Source: three-view drawing plus pictorial views. Frame: mm from the lowest corner of the part. Give positions to 0.01 mm unless a question says otherwise; leave off trailing zeros. Order: outer loops, then holes, each group sorted by start corner. A loop starts at its lowest first (then second) coordinate and runs counter-clockwise, first axis right, second up. Notation, with made-up numbers: (-34.5, 58) - (19.5, 58) arc R9 ccw to (19.5, 72) - close; hole circle Ø3 at (66.5, -13.5). An arc over 180 degrees is marked (long way). Answer in a Markdown table with one row per item. Add a question column.
1. Ray query, line 1 (Y direction, x = 5.25, z = 6); line 2 (Y direction, x = 7.5, z = 7); line 3 (Z direction, x = 6.25, y = 83.75). Return the intervals inside material, ascending. Write a range as [from, to].
2. Contact query for a flat-ended pin moving along its axis: pin 1 (2.5 mm diameter, centred on y = 83.75, z = 6, fed in from +X). Output: stop coordinate, or through.
3. Section query B-B on y = 3.75. Return loops of the section in (x, z), and give its area (3 significant figures).
4. Section query A-A on z = 6. Return loops of the section in (x, y).
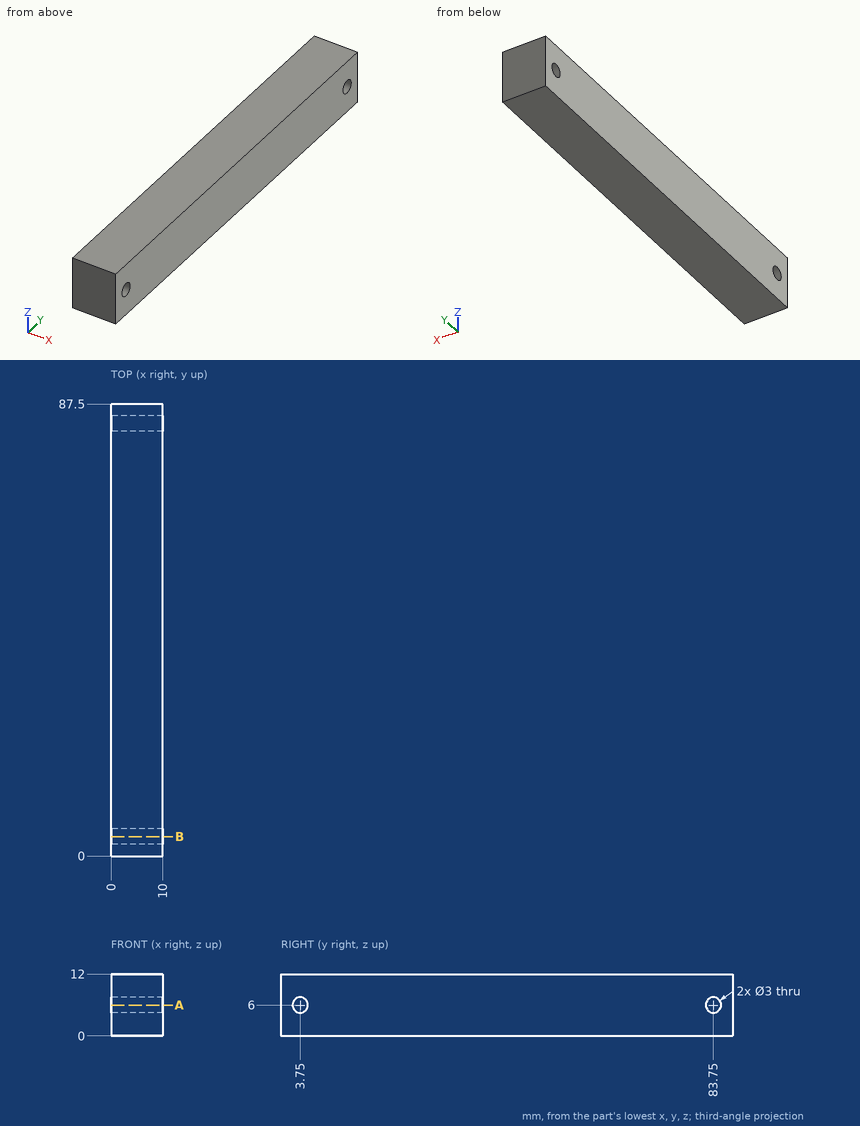
Answer:
| question | item | result |
|---|---|---|
| 1 | line 1 | y = [0, 2.25], [5.25, 82.25], [85.25, 87.5] |
| 1 | line 2 | y = [0, 2.63], [4.87, 82.63], [84.87, 87.5] |
| 1 | line 3 | z = [0, 4.5], [7.5, 12] |
| 2 | pin 1 | passes through |
| 3 | outline | (0, 0) - (10, 0) - (10, 4.5) - (0, 4.5) - close; (0, 7.5) - (10, 7.5) - (10, 12) - (0, 12) - close |
| 3 | area | 90.0 mm² |
| 4 | outline | (0, 0) - (10, 0) - (10, 2.25) - (0, 2.25) - close; (0, 5.25) - (10, 5.25) - (10, 82.25) - (0, 82.25) - close; (0, 85.25) - (10, 85.25) - (10, 87.5) - (0, 87.5) - close |
